Read the model definition and answer for the solid it produces. Units are mm, in the model's axes. Face numbers are marked on the shaded views. A direction names the side the tool comes from. Round coordinates to 2 decimals unless told otherwise and drop trailing zeros. Order: outer loops, then holes, each group sorted by start corner. A loop starts at its lowest first (then second) coordinate and runs counter-clockwise, first axis right, second up. Notation, with made-up numbers: M 25,39.5 L 63,39.5 A14 ccw 63,45.5 Z; hole C -21,53 d2. An arc over 180 degrees is marked long. Answer as CSV lines item,"result".
Autodesk Inventor part; units mm, degrees
ref_plane "YZ Plane" through (0, 0, 0) normal (1, 0, 0) x (0, 1, 0)
ref_plane "XZ Plane" through (0, 0, 0) normal (0, 1, 0) x (-1, 0, 0)
ref_plane "XY Plane" through (0, 0, 0) normal (0, 0, 1) x (1, 0, 0)
sketch "Sketch1" plane through (0, 0, 0) normal (0, 1, 0) x (-1, 0, 0)
  circle A0 centre (0, 0) radius 33.02
  dimension "d0" = 66.04
extrude "Extrusion1" add sketch "Sketch1" along normal blind 2.54
sketch "Sketch2" plane through (0, 2.54, 0) normal (0, 1, 0) x (1, 0, 0)
  circle A0 centre (0, 0) radius 6.35
  dimension "d4" = 12.7
extrude "Extrusion2" add sketch "Sketch2" along normal blind 5.08
fillet "Fillet1" radius 3.175 1 edges at (-6.35, 2.54, 0)
sketch "Sketch3" plane through (0, 7.62, 0) normal (0, 1, 0) x (1, 0, 0)
  circle A0 centre (0, 0) radius 1.6637
  dimension "d8" = 3.3274
extrude "Extrusion3" cut sketch "Sketch3" against normal blind 7.62
fillet "Fillet2" radius 3.175 1 edges at (-6.35, 7.62, 0)
sketch "Sketch4" plane through (0, 0, 0) normal (0, -1, 0) x (1, 0, 0)
  point P0 (0, 0)
sketch "Sketch7" plane through (0, 0, 0) normal (0, -1, 0) x (1, 0, 0)
  circle A0 centre (0, 0) radius 33.02
  arc A1 (32.1408, -7.5691) -> (33.02, 0) centre (0, 0) ccw
  arc A2 (33.02, 0) -> (32.1572, 7.4991) centre (0, 0) ccw
  circle A3 centre (0, 0) radius 1.6637
  line L0 (0, 0) -> (32.6627, -4.8446)
  line L1 (0, 0) -> (32.4709, 5.9969)
  arc A4 (32.6627, -4.8446) -> (32.4709, 5.9969) centre (0, 0) ccw
  line L2 (26.162, -3.8804) -> (26.162, 4.8318)
  arc A5 (32.6627, -4.8446) -> (32.4709, 5.9969) centre (0, 0) ccw
  arc A6 (26.5217, 19.6703) -> (18.7199, 27.2008) centre (0, 0) ccw
  line L3 (0, 0) -> (26.5217, 19.6703)
  line L4 (21.2432, 15.7555) -> (15.0827, 21.9159)
  line L5 (0, 0) -> (18.7199, 27.2008)
  arc A7 (4.8446, 32.6627) -> (-5.9969, 32.4709) centre (0, 0) ccw
  line L6 (0, 0) -> (4.8446, 32.6627)
  line L7 (3.8804, 26.162) -> (-4.8318, 26.162)
  line L8 (0, 0) -> (-5.9969, 32.4709)
  arc A8 (-19.6703, 26.5217) -> (-27.2008, 18.7199) centre (0, 0) ccw
  line L9 (0, 0) -> (-19.6703, 26.5217)
  line L10 (-15.7555, 21.2432) -> (-21.9159, 15.0827)
  line L11 (0, 0) -> (-27.2008, 18.7199)
  arc A9 (-32.6627, 4.8446) -> (-32.4709, -5.9969) centre (0, 0) ccw
  line L12 (0, 0) -> (-32.6627, 4.8446)
  line L13 (-26.162, 3.8804) -> (-26.162, -4.8318)
  line L14 (0, 0) -> (-32.4709, -5.9969)
  arc A10 (-26.5217, -19.6703) -> (-18.7199, -27.2008) centre (0, 0) ccw
  line L15 (0, 0) -> (-26.5217, -19.6703)
  line L16 (-21.2432, -15.7555) -> (-15.0827, -21.9159)
  line L17 (0, 0) -> (-18.7199, -27.2008)
  arc A11 (-4.8446, -32.6627) -> (5.9969, -32.4709) centre (0, 0) ccw
  line L18 (0, 0) -> (-4.8446, -32.6627)
  line L19 (-3.8804, -26.162) -> (4.8318, -26.162)
  line L20 (0, 0) -> (5.9969, -32.4709)
  arc A12 (19.6703, -26.5217) -> (27.2008, -18.7199) centre (0, 0) ccw
  line L21 (0, 0) -> (19.6703, -26.5217)
  line L22 (15.7555, -21.2432) -> (21.9159, -15.0827)
  line L23 (0, 0) -> (27.2008, -18.7199)
  point P0 (23.3487, 23.3487)
  point P1 (0, 33.02)
  point P2 (-23.3487, 23.3487)
  point P3 (-33.02, 0)
  point P4 (-23.3487, -23.3487)
  point P5 (0, -33.02)
  point P6 (23.3487, -23.3487)
  dimension "d25" = 26.162
  dimension "d26" = 8.7122
  dimension "d29" = 360
properties part number "small encoder wheel noah 1"
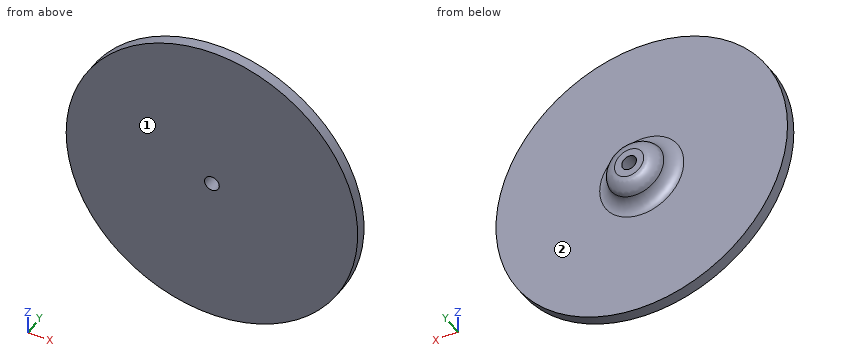
Item 1: Find the intervals of material crossed by probe 1 along Z at (x, y) = (0, 2); probe 2 along X at (y, z) = (3.25, 0); probe 3 along Y at (x, z) = (9, -8), in increasing order. Write a range as [from, to].
Ans:
probe 1,"[-33.02, -1.66], [1.66, 33.02]"
probe 2,"[-7.52, -1.66], [1.66, 7.52]"
probe 3,"[0, 2.54]"
Item 2: A cutting plane is placed at A-A, the plane x = -20. Determine the outline of the cut face in (y, z), and give its area (3 significant figures).
Ans:
outline,"M 0,-26.27 L 2.54,-26.27 L 2.54,26.27 L 0,26.27 Z"
area,"133 mm2"
Item 3: A tool of negligible diameter and unlimited length cuts with its end or side. For the marked faces 1 and 2, from which of +Z, -Z, +X, -X, +Y, -Y can it reach the whole face along a straight path? Write none if from no direction.
Ans:
face 1,"+Z, -Z, +X, -X, -Y"
face 2,"+Y"
Item 4: A cutting plane is placed at B-B, the plane z = 10.5. Determine the outline of the cut face in (x, y).
Ans:
outline,"M -31.31,0 L 31.31,0 L 31.31,2.54 L -31.31,2.54 Z"
Item 5: Flat-ended cylindrical pins translate along their axes: pin 1 (4 mm diameter, centred on x = -7, z = -19.5, fed in from -Y); pin 2 (2 mm diameter, centred on x = 0, z = 0, fed in from +Y); pin 3 (8 mm diameter, centred on x = -14, z = 20.5, fed in from +Y). Find the tip coordinate at first contact, or state that the pin passes through.
Ans:
pin 1,"y = 0"
pin 2,"through"
pin 3,"y = 2.54"
